Can you work these out from the model? Positions are in its coordinate system, mm. A direction names the side the tool comes from. Round coordinates to 2 decimals unless told otherwise and drop trailing zeros. Order: outer loops, then holes, each group sorted by start corner. A loop starts at its lowest first (then second) coordinate and runs counter-clockwise, first axis right, second up. Notation, with made-up numbers: (-29.75, 30.5) -> (19.25, 30.5) arc R17 ccw to (19.25, 39.5) -> close; hole circle Ø4 at (72, 73.5). An arc over 180 degrees is marked (long way). One line per item, written item: value.
```python
from build123d import *

# Parameters (mm, degrees)
F1_DEPTH = 7
F2_W     = 13.5
F2_H     = 2
F3_DEPTH = 4
F5_DEPTH = 22
F6_W     = 13.5
F6_H     = 4
F7_DEPTH = 2


with BuildPart() as f1:
    # F0 (on Front) → F1 (new body)
    with BuildSketch(Plane.XZ):
        Polygon((6.75, -11), (6.75, -9), (6.75, 9), (6.75, 11), (-6.75, 11), (-6.75, 9), (-6.75, -9), (-6.75, -11), align=None)
    extrude(amount=F1_DEPTH)

    # F2 (on face) → F3 (join)
    with BuildSketch(Plane(origin=(0, 0, 0), x_dir=(-1, 0, 0), z_dir=(0, 1, 0))):
        with Locations((0, 6)):
            Rectangle(F2_W, F2_H)
    extrude(amount=F3_DEPTH)

    # F4 (on face) → F5 (cut, through all)
    with BuildSketch(Plane.XY.offset(11)):
        Polygon((4, -7), (0, -3), (-4, -7), align=None)
    extrude(amount=-F5_DEPTH, mode=Mode.SUBTRACT)

    # F6 (on face) → F7 (cut)
    with BuildSketch(Plane(origin=(0, 0, 0), x_dir=(-1, 0, 0), z_dir=(0, 1, 0))):
        with Locations((0, 1)):
            Rectangle(F6_W, F6_H)
        with Locations((0, -7)):
            Rectangle(F6_W, F6_H)
    extrude(amount=-F7_DEPTH, mode=Mode.SUBTRACT)


solid = f1.part
```
Q1. We'd pull the mould along Z, two halves only. Please class faces 1 (the face through (0, -1, -9)), 2 (the face through (0, -2, -7)), 3 (the face through (0, 0, -3)), 4 (the face through (0, 2, 5)): released by +Z, released by -Z, zero draft, split by the parting line, or undercut.
Answers below:
face 1: undercut
face 2: undercut
face 3: zero draft
face 4: released by -Z
Q2. I want a section at D-D on x = -4.75. List the corners of the cut face in (y, z) for me.
Answers below:
outline: (-7, -11) -> (0, -11) -> (0, -9) -> (-2, -9) -> (-2, -5) -> (0, -5) -> (0, -1) -> (-2, -1) -> (-2, 3) -> (0, 3) -> (0, 5) -> (4, 5) -> (4, 7) -> (0, 7) -> (0, 11) -> (-7, 11) -> close
Q3. Will these pins go through, and if not, where does the flat tip stop? pin 1 Ø1 at (x, z) = (4, -2.5) entering from +Y; pin 2 Ø4.5 at (x, y) = (-2.5, 3) entering from -Z; pin 3 Ø3 at (x, z) = (-2, 1.5) entering from -Y.
Answers below:
pin 1: y = 0
pin 2: z = 5
pin 3: y = -6.5
Q4. I want a section at B-B on x = 0.5. List the corners of the cut face in (y, z) for me.
Answers below:
outline: (-3.5, -11) -> (0, -11) -> (0, -9) -> (-2, -9) -> (-2, -5) -> (0, -5) -> (0, -1) -> (-2, -1) -> (-2, 3) -> (0, 3) -> (0, 5) -> (4, 5) -> (4, 7) -> (0, 7) -> (0, 11) -> (-3.5, 11) -> close
Q5. I want a section at C-C on z = -1.5. List the corners of the cut face in (x, y) for me.
Answers below:
outline: (-6.75, -7) -> (-4, -7) -> (0, -3) -> (4, -7) -> (6.75, -7) -> (6.75, 0) -> (-6.75, 0) -> close
Q6. Please list where these lines run through material, in increasing order: line 1 along Z through (x, y) = (-1.75, -1); line 2 along Y through (x, z) = (6, -2); line 3 along X through (y, z) = (-6.5, 10).
Answers below:
line 1: -11 to -9, -5 to -1, 3 to 11
line 2: -7 to 0
line 3: -6.75 to -3.5, 3.5 to 6.75
Q7. On a 3-axis mill with a long thin cutter (end or side, diameter ignored), from which of +Z, -Z, +X, -X, +Y, -Y can I reach the whole of each face in a straight line? I mean faces 5 (the face through (0, -1, -5)), 6 (the face through (0, 0, 9)), 7 (the face through (0, 0, -10)), 8 (the face through (-2, -5, 0)). Say none if no direction works.
Answers below:
face 5: +X, -X, +Y
face 6: +Z, +X, -X, +Y
face 7: -Z, +X, -X, +Y
face 8: +Z, -Z, -Y
Q8. I want a section at A-A on y = -4.75. List the corners of the cut face in (x, z) for me.
Answers below:
outline: (-6.75, -11) -> (-1.75, -11) -> (-1.75, 11) -> (-6.75, 11) -> close; (1.75, -11) -> (6.75, -11) -> (6.75, 11) -> (1.75, 11) -> close
